Design review of the part built by this model. Coordinates are the model's own, in mm. A direction names the side the tool comes from. Give positions to 0.01 mm unless a question says otherwise; leave off trailing zeros. Write each loop counter-clockwise with the first axis right and the second up, starting at its lowest first coordinate (ties: lowest second). Pieces come first, ordered by that corner, then holes. Notation, with made-up numbers: (72, 34) - (106, 34) arc R16 ccw to (106, 65) - close; hole circle Ø6 at (-31.5, -9.5). An arc over 180 degrees is marked (long way). Use a Markdown table: item, result. Add a question column.
Autodesk Inventor part; units mm, degrees
ref_plane "YZ Plane" through (0, 0, 0) normal (1, 0, 0) x (0, 1, 0)
ref_plane "XZ Plane" through (0, 0, 0) normal (0, 1, 0) x (-1, 0, 0)
ref_plane "XY Plane" through (0, 0, 0) normal (0, 0, 1) x (1, 0, 0)
sketch "Sketch1" plane through (0, 0, 0) normal (1, 0, 0) x (0, 1, 0)
  line L0 (15.5, -16) -> (-15.5, -16)
  line L1 (-15.5, -16) -> (-15.5, 16)
  line L2 (-15.5, 16) -> (15.5, 16)
  line L3 (15.5, 16) -> (15.5, -16)
  line L4 (15.5, -16) -> (-15.5, 16) construction
  line L5 (-15.5, -16) -> (15.5, 16) construction
  line L6 (-8.37, 8) -> (-8.37, -8) construction
  line L7 (-6.22, 8) -> (-6.22, -8)
  line L8 (-10.52, -8) -> (-10.52, 8)
  arc A0 (-6.22, 8) -> (-10.52, 8) centre (-8.37, 8) ccw
  arc A1 (-10.52, -8) -> (-6.22, -8) centre (-8.37, -8) ccw
  point P0 (0, 0)
  point P1 (-8.37, 0)
  dimension "d0" = 31
  dimension "d1" = 32
  dimension "d5" = 7.13
  dimension "d6" = 16
  dimension "d7" = 4.3
extrude "Extrusion1" add sketch "Sketch1" along normal blind 2
fillet "Fillet1" radius 0.5 4 edges at (1, 15.5, 16) (1, -15.5, 16) (1, -15.5, -16) (1, 15.5, -16)
properties part number "3DPRINT,LIMIT_SWITCH,SPACER" material "ABS Plastic"
(1) Add section C-C (x = 1.7). State the section outline as (y, z) points, and give its area (3 significant figures).
(2) For line 1 along Y through (x, z) = (0.6, -1); line 2 along Z through (x, y) = (0.95, -8); line 3 along Z through (x, y) = (1.6, -10), list the stretches that pass through material, from the lowest coordinate up.
(3) Mouldability with a two-part tool opening along Z and no side actions: class faces 1 (the face through (1, 0, -16)), 2 (the face through (1, -15.5, 0)), 3 (the face through (1, -6.22, 0)), 4 (the face through (0.99, -8.42, 10.15)) as +Z half, -Z half, draft (parallel to the pull), parting line (faces both ways), or undercut.
(4) Tool access review of faces 5 (the face through (2, 0, 0)), 6 (the face through (1, -10.52, 0)): name each direction out of +Z, -Z, +X, -X, +Y, -Y from which nothing blocks a thin tool from reaching the whole face with its end or side.
(5) Add section B-B (z = -0.5). State the section outline as (x, y) points.
(6) Add section A-A (y = -8.37). State the section outline as (x, z) points, and give its area (3 significant figures).
Answers follow:
| question | item | result |
|---|---|---|
| 1 | outline | (-15.5, -15.5) arc R0.5 ccw to (-15, -16) - (15, -16) arc R0.5 ccw to (15.5, -15.5) - (15.5, 15.5) arc R0.5 ccw to (15, 16) - (-15, 16) arc R0.5 ccw to (-15.5, 15.5) - close; hole (-10.52, -8) arc R2.15 ccw to (-6.22, -8) - (-6.22, 8) arc R2.15 ccw to (-10.52, 8) - close |
| 1 | area | 908 mm^2 |
| 2 | line 1 | -15.5 to -10.52, -6.22 to 15.5 |
| 2 | line 2 | -16 to -10.12, 10.12 to 16 |
| 2 | line 3 | -16 to -9.4, 9.4 to 16 |
| 3 | face 1 | -Z half |
| 3 | face 2 | draft |
| 3 | face 3 | undercut |
| 3 | face 4 | undercut |
| 4 | face 5 | +Z, -Z, +X, +Y, -Y |
| 4 | face 6 | +X, -X |
| 5 | outline | (0, -15.5) - (2, -15.5) - (2, -10.52) - (0, -10.52) - close; (0, -6.22) - (2, -6.22) - (2, 15.5) - (0, 15.5) - close |
| 6 | outline | (0, -16) - (2, -16) - (2, -10.15) - (0, -10.15) - close; (0, 10.15) - (2, 10.15) - (2, 16) - (0, 16) - close |
| 6 | area | 23.4 mm^2 |
